For this review, take the finished solid that the model builds, in its own axes (mm). Face numbers are marked on the shaded views. Give positions to 0.01 mm unless a question says otherwise; leave off trailing zeros. Loops run counter-clockwise (first coordinate to the right, second up) from the corner with the lowest first, then second, coordinate; pieces in that order, holes last. Notation, with made-up numbers: (42, 59.5) - (63, 59.5) arc R15 cw to (63, 75.5) - close; hole circle Ø8 at (1.5, 64.5). An arc over 180 degrees is marked (long way). Answer as CSV lines item,"result".
from build123d import *

# Parameters (mm, degrees)
SKETCH1_R           = 40
SKETCH1_R_2         = 25
BOSS_EXTRUDE1_DEPTH = 50
SKETCH2_R           = 2.1
CUT_EXTRUDE1_DEPTH  = 10
BOSS_EXTRUDE2_START = -50
BOSS_EXTRUDE2_DEPTH = 12
BOSS_EXTRUDE3_START = -7
SKETCH4_R           = 15
SKETCH4_R_2         = 11.1
BOSS_EXTRUDE3_DEPTH = 7
BOSS_EXTRUDE4_START = 10
SKETCH5_R           = 15
SKETCH5_R_2         = 9
BOSS_EXTRUDE4_DEPTH = 10
BOSS_EXTRUDE5_START = 7
SKETCH6_R           = 15
SKETCH6_R_2         = 11.1
BOSS_EXTRUDE5_DEPTH = 7
FILLET1_R           = 2


with BuildPart() as part:
    # Sketch1 → Boss-Extrude1 (new, symmetric)
    with BuildSketch(Plane(origin=(0, 0, 0), x_dir=(1, 0, 0), z_dir=(0, 1, 0))):
        with Locations(Location((0, 0, 0), (0, 0, 90))):
            Circle(SKETCH1_R)
        with Locations(Location((0, 0, 0), (0, 0, 90))):
            Circle(SKETCH1_R_2, mode=Mode.SUBTRACT)
    extrude(amount=BOSS_EXTRUDE1_DEPTH, both=True)

    # Sketch2 → Cut-Extrude1 (cut)
    with BuildSketch(Plane(origin=(0, 50, 0), x_dir=(1, 0, 0), z_dir=(0, 1, 0))):
        with Locations(Location((0, 35, 0), (0, 0, 270))):
            Circle(SKETCH2_R)
        with Locations(Location((35, 0, 0), (0, 0, 270))):
            Circle(SKETCH2_R)
        with Locations(Location((0, -35, 0), (0, 0, 270))):
            Circle(SKETCH2_R)
        with Locations(Location((-35, 0, 0), (0, 0, 270))):
            Circle(SKETCH2_R)
    cut_extrude1 = extrude(amount=-CUT_EXTRUDE1_DEPTH, mode=Mode.SUBTRACT)

    # Mirror1: Cut-Extrude1 across plane
    add(cut_extrude1.mirror(Plane.ZX), mode=Mode.SUBTRACT)

    # Sketch3 → Boss-Extrude2 (add, symmetric)
    with BuildSketch(Plane.XZ.offset(50).offset(BOSS_EXTRUDE2_START)):
        with BuildLine():
            ThreePointArc((-2.604722665, 14.772116295), (-1.307336141, 14.942920471), (0, 15))
            Line((0, 15), (0, 25))
            ThreePointArc((0, 25), (-2.178893569, 24.904867452), (-4.341204442, 24.620193825))
            Line((-4.341204442, 24.620193825), (-2.604722665, 14.772116295))
        make_face()
        with BuildLine():
            Line((0, 25), (0, 15))
            ThreePointArc((0, 15), (1.307336141, 14.942920471), (2.604722665, 14.772116295))
            Line((2.604722665, 14.772116295), (4.341204442, 24.620193825))
            ThreePointArc((4.341204442, 24.620193825), (2.178893569, 24.904867452), (0, 25))
        make_face()
    boss_extrude2 = extrude(amount=BOSS_EXTRUDE2_DEPTH, both=True)

    # Mirror2: Boss-Extrude2 across plane
    add(boss_extrude2.mirror(Plane.XY))

    # Sketch4 → Boss-Extrude3 (add)
    with BuildSketch(Plane(origin=(0, 12, 0), x_dir=(1, 0, 0), z_dir=(0, 1, 0)).offset(BOSS_EXTRUDE3_START)):
        Circle(SKETCH4_R)
        with Locations(Location((0, 0, 0), (0, 0, 270))):
            Circle(SKETCH4_R_2, mode=Mode.SUBTRACT)
    extrude(amount=BOSS_EXTRUDE3_DEPTH)

    # Sketch5 → Boss-Extrude4 (add)
    with BuildSketch(Plane.XZ.offset(-5).offset(BOSS_EXTRUDE4_START)):
        Circle(SKETCH5_R)
        with Locations(Location((0, 0, 0), (0, 0, 270))):
            Circle(SKETCH5_R_2, mode=Mode.SUBTRACT)
    extrude(amount=-BOSS_EXTRUDE4_DEPTH)

    # Sketch6 → Boss-Extrude5 (add)
    with BuildSketch(Plane.XZ.offset(5).offset(BOSS_EXTRUDE5_START)):
        Circle(SKETCH6_R)
        with Locations(Location((0, 0, 0), (0, 0, 90))):
            Circle(SKETCH6_R_2, mode=Mode.SUBTRACT)
    extrude(amount=-BOSS_EXTRUDE5_DEPTH)

    # Fillet1
    fillet1_edges = [part.edges().sort_by_distance(p)[0] for p in [
        (2.604722665, 0, 14.772116295),
        (-2.604722665, 0, 14.772116295),
        (-4.341204442, 0, 24.620193825),
        (4.341204442, 0, 24.620193825),
        (-2.604722665, 0, -14.772116295),
        (2.604722665, 0, -14.772116295),
        (4.341204442, 0, -24.620193825),
        (-4.341204442, 0, -24.620193825),
    ]]
    fillet(fillet1_edges, radius=FILLET1_R)


solid = part.part
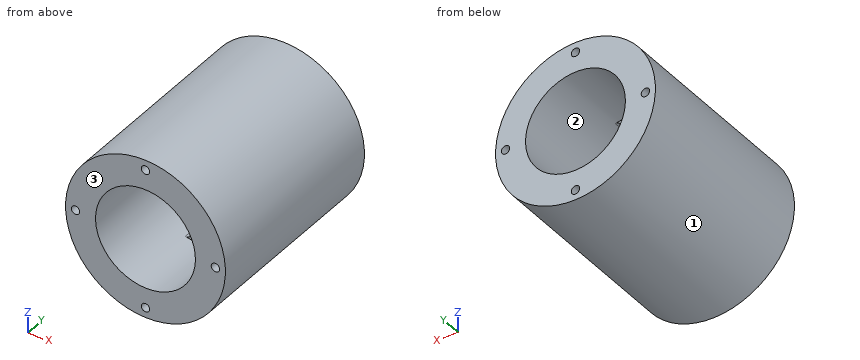
1) Draft analysis for pull direction X (two halves, no side actions). For the marked faces 1, 2 and 3, state which applies: pulls with the +X half, pulls with the -X half, needs draft (parallel to the pull), parting line crosses it, or undercut.
From the geometry:
face 1,"parting line crosses it"
face 2,"undercut"
face 3,"needs draft"
2) Wall thickness on line 1 (X direction, y = 43.5, z = 0); line 2 (X direction, y = -8.5, z = -20.5); line 3 (Z direction, x = 8.5, y = -21): over which ranges is each line inside the solid? List them lowest first. Write a range as from..to.
From the geometry:
line 1,"x = -40..-37.1, -32.9..-25, 25..32.9, 37.1..40"
line 2,"x = -34.35..-14.31, -3.61..3.61, 14.31..34.35"
line 3,"z = -39.09..-23.51, 23.51..39.09"
3) Consider section B-B on y = -25. Write out the cut boundary in (x, z).
From the geometry:
outline,"circle Ø80 at (0, 0); hole circle Ø50 at (0, 0)"
4) Consider section C-C on y = 0. Write out the cut boundary in (x, z).
From the geometry:
outline,"circle Ø80 at (0, 0); hole circle Ø18 at (0, 0); hole (-6.47, -24.15) arc R2 ccw to (-3.98, -22.56) - (-2.93, -16.63) arc R2 ccw to (-4.32, -14.36) arc R15 cw to (-4.32, 14.36) arc R2 ccw to (-2.93, 16.63) - (-3.98, 22.56) arc R2 ccw to (-6.47, 24.15) arc R25 ccw to start; hole (2.93, -16.63) - (3.98, -22.56) arc R2 ccw to (6.47, -24.15) arc R25 ccw to (6.47, 24.15) arc R2 ccw to (3.98, 22.56) - (2.93, 16.63) arc R2 ccw to (4.32, 14.36) arc R15 cw to (4.32, -14.36) arc R2 ccw to start"
5) Consider section A-A on x = -23. Write out the cut boundary in (y, z), and give its area (3 significant figures).
From the geometry:
outline,"(-50, -32.73) - (50, -32.73) - (50, -9.8) - (-50, -9.8) - close; (-50, 9.8) - (50, 9.8) - (50, 32.73) - (-50, 32.73) - close"
area,"4,590 mm^2"
6) Consider section D-D on z = 0. Count the separate pieces of the cut face and the enclosed holes in it, and give its area (3 significant figures).
From the geometry:
separate pieces,"4"
enclosed holes,"0"
area,"3,060 mm^2"
7) Insertion check: P1, Ø2, axis at x = 34, z = 0, coming from the -Y side; P2, Ø5, axis at x = 26, y = 32.5, coming from the -Z side; P3, Ø5, axis at y = -19, z = 28, coming from the +X side. Each pin has a flat end and moves straight along its axis. Give the tip position at first contact, or say it passes through.
From the geometry:
P1,"stops at y = -40"
P2,"stops at z = -32.37"
P3,"stops at x = 30.82"
